from build123d import *

# Parameters (mm, degrees)
BOSS_EXTRUDE1_DEPTH     = 2
SKETCH2_R               = 1.375
CUT_EXTRUDE1_DEPTH      = 2
CUT_EXTRUDE3_DEPTH      = 47.745974282
CUT_EXTRUDE3_DEPTH_BACK = 47.745974282
SKETCH12_R              = 1.375
BOSS_EXTRUDE2_START     = -1.875
BOSS_EXTRUDE2_DEPTH     = 7.715
SKETCH16_R              = 1.375
BOSS_EXTRUDE3_DEPTH     = 3.086
LPATTERN1_COUNT         = 3
LPATTERN1_PITCH         = 6.172


with BuildPart() as part:
    # Sketch1 → Boss-Extrude1 (new body)
    with BuildSketch(Plane(origin=(0, 0, 0), x_dir=(1, 0, 0), z_dir=(0, 1, 0))):
        with BuildLine():
            Line((-6.5, 0), (6.5, 0))
            Line((6.5, 0), (6.5, 5.19))
            add(Edge.make_bspline(
                [(-6.5, 5.19), (0, 3.63), (6.5, 5.19)],
                knots=[0, 0, 0, 1, 1, 1], degree=2))
            Line((-6.5, 5.19), (-6.5, 0))
        make_face()
    extrude(amount=BOSS_EXTRUDE1_DEPTH)

    # Sketch2 → Cut-Extrude1 (cut)
    with BuildSketch(Plane(origin=(0, 2, 0), x_dir=(1, 0, 0), z_dir=(0, 1, 0))):
        with Locations(Location((-4, 2.595, 0), (0, 0, 270))):
            Circle(SKETCH2_R)
        with Locations(Location((4, 2.595, 0), (0, 0, 270))):
            Circle(SKETCH2_R)
    extrude(amount=-CUT_EXTRUDE1_DEPTH, mode=Mode.SUBTRACT)

    # Sketch4 → Loft2 section 0
    with BuildSketch(Plane(origin=(0, 2, 0), x_dir=(1, 0, 0), z_dir=(0, 1, 0))):
        with BuildLine():
            Line((-1.875, 3.75), (1.875, 3.75))
            Line((1.875, 3.75), (1.875, 0))
            Line((1.875, 0), (-1.875, 0))
            Line((-1.875, 0), (-1.875, 3.75))
        make_face()
    # Sketch6 → Loft2 section 1
    with BuildSketch(Plane(origin=(0, 46, 0), x_dir=(1, 0, 0), z_dir=(0, 1, 0))):
        with BuildLine():
            Line((-1.875, 1), (1.875, 1))
            Line((1.875, 1), (1.875, -2.75))
            Line((1.875, -2.75), (-1.875, -2.75))
            Line((-1.875, -2.75), (-1.875, 1))
        make_face()
    loft()

    # Sketch12 → Cut-Extrude3 (cut, two sides: drawn at the far end of the back side and taken through both)
    with BuildSketch(Plane.XY.offset(-CUT_EXTRUDE3_DEPTH_BACK)):
        with Locations(Location((0, 44, 0), (0, 0, 90))):
            Circle(SKETCH12_R)
    extrude(amount=CUT_EXTRUDE3_DEPTH + CUT_EXTRUDE3_DEPTH_BACK, mode=Mode.SUBTRACT)

    # Sketch13 → Boss-Extrude2 (add)
    with BuildSketch(Plane.ZY.offset(1.875).offset(BOSS_EXTRUDE2_START)):
        Polygon((-3.398125, 13.63), (-3.398125, 7.63), (0.351875, 7.63), (0.726875, 13.63), align=None)
    boss_extrude2 = extrude(amount=BOSS_EXTRUDE2_DEPTH)

    # Mirror1: Boss-Extrude2 across plane
    add(boss_extrude2.mirror(Plane(origin=(0, 0, 0), x_dir=(0, 0, 1), z_dir=(1, 0, 0))))

    # Sketch16 → Boss-Extrude3 (add)
    with BuildSketch(Plane.ZY.offset(7.715)):
        with BuildLine():
            Line((-3.398125, 7.63), (-6.798125, 7.63))
            ThreePointArc((-6.798125, 7.63), (-9.798125, 10.63), (-6.798125, 13.63))
            Line((-6.798125, 13.63), (-3.398125, 13.63))
            Line((-3.398125, 13.63), (-3.398125, 7.63))
        make_face()
        with Locations((-6.798125, 10.63)):
            Circle(SKETCH16_R, mode=Mode.SUBTRACT)
    boss_extrude3 = extrude(amount=-BOSS_EXTRUDE3_DEPTH)

    # LPattern1: Boss-Extrude3 ×3
    with Locations(*[(i * LPATTERN1_PITCH, 0, 0) for i in range(1, LPATTERN1_COUNT)]):
        add(boss_extrude3)


solid = part.part
The listing builds one solid part. Answer for the finished solid, in the listing's coordinates (mm). A direction names the side the tool comes from. Coordinates: 2 decimals unless noted, no trailing zeros. Order: outer loops, then holes, each group sorted by start corner. A loop starts at its lowest first (then second) coordinate and runs counter-clockwise, first axis right, second up. Notation, with made-up numbers: (58, 4) -> (90, 4) arc R13 cw to (90, 29) -> close; hole circle Ø1 at (-28, -6.75). An arc over 180 degrees is marked (long way). Answer in a Markdown table with one row per item. Add a question column.
Item 1: Find section A-A (x = 0). State how many separate pieces and enclosed holes the cut face has, then the cut area to 3 significant figures.
Item 2: Find section B-B (z = -7.5). Write down the section's boundary in (x, y) (3 decimals).
Item 3: Find section C-C (y = 10.63). Write down the section's boundary in (x, z) (3 decimals).
Item 4: Find the intervals of material crossed by L1, parallel to X at y = 13, z = -4.25 (3 decimals); L2, parallel to Y at x = 6.75, z = -6.75; L3, parallel to Y at x = -2.5, z = -1.5, in increasing order. Write a range as from..to.
Item 5: Which of the six approach directions +Z, -Z, +X, -X, +Y, -Y give full straight-line access (tool end or side, diameter ignored) to faces 1 (the face through (1.543, 11, -5)), 2 (the face through (-0.03, 4.85, -3.57)), 3 (the face through (0, 1, 0))?
Item 6: Determine the mould class of faces 4 (the face through (6.5, 1, -3)), 5 (the face through (0, 30, -2)), 6 (the face through (-4.527, 1.014, -1.325)), 7 (the face through (3, 11, -3.398)) for opening direction X: +X half, -X half, draft (parallel to the pull), parting line (faces both ways), or undercut.
Item 7: Each of these flat-tipped pins is pushed along its axis until it touches: P1, Ø8, axis at x = 0, y = 8.5, coming from the +Z side; P2, Ø0.9, axis at x = 0.5, z = -6, coming from the -Y side; P3, Ø5, axis at y = 18.5, z = -3, coming from the +X side (3 decimals). Where does it stop, or does it pass through?
Result set:
| question | item | result |
|---|---|---|
| 1 | separate pieces | 2 |
| 1 | enclosed holes | 1 |
| 1 | area | 193 mm² |
| 2 | outline | (-7.715, 7.713) -> (-4.629, 7.713) -> (-4.629, 9.448) -> (-7.715, 9.448) -> close; (-7.715, 11.812) -> (-4.629, 11.812) -> (-4.629, 13.547) -> (-7.715, 13.547) -> close; (-1.543, 7.713) -> (1.543, 7.713) -> (1.543, 9.448) -> (-1.543, 9.448) -> close; (-1.543, 11.812) -> (1.543, 11.812) -> (1.543, 13.547) -> (-1.543, 13.547) -> close; (4.629, 7.713) -> (7.715, 7.713) -> (7.715, 9.448) -> (4.629, 9.448) -> close; (4.629, 11.812) -> (7.715, 11.812) -> (7.715, 13.547) -> (4.629, 13.547) -> close |
| 3 | outline | (-7.715, -9.798) -> (-4.629, -9.798) -> (-4.629, -8.173) -> (-7.715, -8.173) -> close; (-7.715, -5.423) -> (-4.629, -5.423) -> (-4.629, -3.398) -> (-1.543, -3.398) -> (-1.543, -5.423) -> (1.543, -5.423) -> (1.543, -3.398) -> (4.629, -3.398) -> (4.629, -5.423) -> (7.715, -5.423) -> (7.715, 0.539) -> (-7.715, 0.539) -> close; (-1.543, -9.798) -> (1.543, -9.798) -> (1.543, -8.173) -> (-1.543, -8.173) -> close; (4.629, -9.798) -> (7.715, -9.798) -> (7.715, -8.173) -> (4.629, -8.173) -> close |
| 4 | L1 | x = -7.715..-4.629, -1.543..1.543, 4.629..7.715 |
| 4 | L2 | y = 7.63..9.26, 12..13.63 |
| 4 | L3 | y = 0..2, 7.63..13.63 |
| 5 | face 1 | -Z, +Y |
| 5 | face 2 | -Z, +X, -X |
| 5 | face 3 | +Z, +X, -X, -Y |
| 6 | face 4 | +X half |
| 6 | face 5 | draft |
| 6 | face 6 | undercut |
| 6 | face 7 | undercut |
| 7 | P1 | stops at z = 0.66 |
| 7 | P2 | stops at y = 7.63 |
| 7 | P3 | stops at x = 1.875 |
